Can you work these out from the model? Positions are in its coordinate system, mm. A direction names the side the tool comes from. Coordinates: 2 decimals unless noted, no trailing zeros. Write each loop counter-clockwise with the first axis right and the second up, starting at its lowest first coordinate (ties: lowest second). Pieces come first, ordered by that corner, then holes. Notation, with made-up numbers: (80, 82) -> (117, 82) arc R32 ccw to (117, 116) -> close; hole circle Ø7 at (-17, 65.5). An arc over 180 degrees is marked (long way). Use one line per item in the form item = value.
```python
from build123d import *

# Parameters (mm, degrees)
SKIZZE1_W                       = 28
SKIZZE1_H                       = 47
AUFSATZ_LINEAR_AUSTRAGEN1_DEPTH = 12
SCHNITT_LINEAR_AUSTRAGEN1_DEPTH = 9.5
VERRUNDUNG2_R                   = 1
SKIZZE3_R                       = 0.5
SCHNITT_LINEAR_AUSTRAGEN2_DEPTH = 3


with BuildPart() as part:
    # Skizze1 → Aufsatz-Linear austragen1 (new body)
    with BuildSketch(Plane.XY):
        with Locations((14, 23.5)):
            Rectangle(SKIZZE1_W, SKIZZE1_H)
    extrude(amount=AUFSATZ_LINEAR_AUSTRAGEN1_DEPTH)

    # Skizze2 → Schnitt-Linear austragen1 (cut)
    with BuildSketch(Plane.XY.offset(12)):
        with BuildLine():
            Line((2.5, 45.5), (25.5, 45.5))
            ThreePointArc((25.5, 45.5), (26.207106781, 45.207106781), (26.5, 44.5))
            Line((26.5, 44.5), (26.5, 8.251904421))
            Line((26.5, 8.251904421), (25.5, 7.5))
            Line((25.5, 7.5), (25.5, 5.5))
            Line((25.5, 5.5), (26.5, 4.751904421))
            Line((26.5, 4.751904421), (26.5, 1.5))
            Line((26.5, 1.5), (26, 1.5))
            Line((26, 1.5), (26, 0))
            Line((26, 0), (2, 0))
            Line((2, 0), (2, 1.5))
            Line((2, 1.5), (1.5, 1.5))
            Line((1.5, 1.5), (1.5, 4.751904421))
            Line((1.5, 4.751904421), (2.5, 5.5))
            Line((2.5, 5.5), (2.5, 7.5))
            Line((2.5, 7.5), (1.5, 8.251904421))
            Line((1.5, 8.251904421), (1.5, 44.5))
            ThreePointArc((1.5, 44.5), (1.792893219, 45.207106781), (2.5, 45.5))
        make_face()
    extrude(amount=-SCHNITT_LINEAR_AUSTRAGEN1_DEPTH, mode=Mode.SUBTRACT)

    # Verrundung2
    verrundung2_edges = [part.edges().sort_by_distance(p)[0] for p in [
        (0, 47, 6),
        (28, 47, 6),
    ]]
    fillet(verrundung2_edges, radius=VERRUNDUNG2_R)

    # Skizze3 → Schnitt-Linear austragen2 (cut)
    with BuildSketch(Plane.XY.offset(12)):
        with Locations((1.1, 45.9)):
            Circle(SKIZZE3_R)
        with Locations((26.9, 45.9)):
            Circle(SKIZZE3_R)
        with Locations((0.9, 0.8)):
            Circle(SKIZZE3_R)
        with Locations((27.1, 0.8)):
            Circle(SKIZZE3_R)
    extrude(amount=-SCHNITT_LINEAR_AUSTRAGEN2_DEPTH, mode=Mode.SUBTRACT)


solid = part.part
```
Q1. Suppose I cut it at C-C (x = 4.75). Write out the boundary of the cut face in (y, z), then the cut area to 3 significant figures.
Return value:
outline = (0, 0) -> (47, 0) -> (47, 12) -> (45.5, 12) -> (45.5, 2.5) -> (0, 2.5) -> close
area = 132 mm2
Q2. If I drill on line 1 (X direction, y = 45.9, z = 10.65); line 2 (X direction, y = 26, z = 6.75); line 3 (Y direction, x = 26.9, z = 10.05), over which ranges is the centre line in solid material (lowest first)? Write a range as from..to.
Return value:
line_1 = 0..0.6, 1.6..26.4, 27.4..28
line_2 = 0..1.5, 26.5..28
line_3 = 0..0.34, 1.26..45.4, 46.4..47
Q3. Suppose I cut it at B-B (y = 30.5). Write out the boundary of the cut face in (x, z), then the cut area to 3 significant figures.
Return value:
outline = (0, 0) -> (28, 0) -> (28, 12) -> (26.5, 12) -> (26.5, 2.5) -> (1.5, 2.5) -> (1.5, 12) -> (0, 12) -> close
area = 98.5 mm2
Q4. For faces 1 (the flat face through (26, 1, 7)), 2 (the cylindrical face through (0.5, 0.5, 10.5)), 3 (the flat face through (0, 23, 6)), which set-ups out of +Z, -Z, +X, -X, +Y, -Y let a thin tool reach every point of the face, with its end or its side?
Return value:
face_1 = +Z, -Y
face_2 = +Z
face_3 = +Z, -Z, -X, +Y, -Y
Q5. Suppose I cut it at A-A (z = 3.5). Write out the boundary of the cut face in (x, y).
Return value:
outline = (0, 0) -> (2, 0) -> (2, 1.5) -> (1.5, 1.5) -> (1.5, 4.75) -> (2.5, 5.5) -> (2.5, 7.5) -> (1.5, 8.25) -> (1.5, 44.5) arc R1 cw to (2.5, 45.5) -> (25.5, 45.5) arc R1 cw to (26.5, 44.5) -> (26.5, 8.25) -> (25.5, 7.5) -> (25.5, 5.5) -> (26.5, 4.75) -> (26.5, 1.5) -> (26, 1.5) -> (26, 0) -> (28, 0) -> (28, 46) arc R1 ccw to (27, 47) -> (1, 47) arc R1 ccw to (0, 46) -> close
Q6. Will this pin go through, and if not, where does the flat tip stop? pin 1 (5 mm diameter, centred on x = 20.5, y = 7, fed in from +Z).
Return value:
pin_1 = 2.5
Q7. Suppose I cut it at D-D (y = 0.8). Write out the boundary of the cut face in (x, z), then the cut area to 3 significant figures.
Return value:
outline = (0, 0) -> (28, 0) -> (28, 12) -> (27.6, 12) -> (27.6, 9) -> (26.6, 9) -> (26.6, 12) -> (26, 12) -> (26, 2.5) -> (2, 2.5) -> (2, 12) -> (1.4, 12) -> (1.4, 9) -> (0.4, 9) -> (0.4, 12) -> (0, 12) -> close
area = 102 mm2
